Can you work these out from the model? Positions are in its coordinate system, mm. Face numbers are marked on the shaded views. Coordinates: 2 decimals unless noted, no trailing zeros. Loops run counter-clockwise (first coordinate to the right, second up) from the corner with the lowest first, then second, coordinate; pieces in that order, holes last. Notation, with made-up numbers: (37.5, 72) - (46.5, 72) arc R25 ccw to (46.5, 96) - close; hole circle Ø6 at (55, 32). An arc over 180 degrees is marked (long way). Put each result on its own line as item: value. Start each with the question number.
from build123d import *

# Parameters (mm, degrees)
SKETCH1_W           = 76.2
SKETCH1_H           = 31.75
BOSS_EXTRUDE1_DEPTH = 1.27
FILLET1_R           = 3.175
SKETCH2_W           = 68.58
SKETCH2_H           = 24.13
BOSS_EXTRUDE2_DEPTH = 1.27
SKETCH3_R           = 1.27
CUT_EXTRUDE1_DEPTH  = 42.353079994
CHAMFER1_SIZE       = 0.508


with BuildPart() as part:
    # Sketch1 → Boss-Extrude1 (new body)
    with BuildSketch(Plane(origin=(0, 0, 0), x_dir=(1, 0, 0), z_dir=(0, 1, 0))):
        Rectangle(SKETCH1_W, SKETCH1_H)
    extrude(amount=BOSS_EXTRUDE1_DEPTH)

    # Fillet1
    fillet1_edges = [part.edges().sort_by_distance(p)[0] for p in [
        (-38.1, 0.635, -15.875),
        (38.1, 0.635, -15.875),
        (38.1, 0.635, 15.875),
        (-38.1, 0.635, 15.875),
    ]]
    fillet(fillet1_edges, radius=FILLET1_R)

    # Sketch2 → Boss-Extrude2 (add)
    with BuildSketch(Plane(origin=(0, 1.27, 0), x_dir=(1, 0, 0), z_dir=(0, 1, 0))):
        with BuildLine():
            Line((34.925, 13.335), (-34.925, 13.335))
            ThreePointArc((-34.925, 13.335), (-35.374012806, 13.149012806), (-35.56, 12.7))
            Line((-35.56, 12.7), (-35.56, -12.7))
            ThreePointArc((-35.56, -12.7), (-35.374012806, -13.149012806), (-34.925, -13.335))
            Line((-34.925, -13.335), (34.925, -13.335))
            ThreePointArc((34.925, -13.335), (35.374012806, -13.149012806), (35.56, -12.7))
            Line((35.56, -12.7), (35.56, 12.7))
            ThreePointArc((35.56, 12.7), (35.374012806, 13.149012806), (34.925, 13.335))
        make_face()
        Rectangle(SKETCH2_W, SKETCH2_H, mode=Mode.SUBTRACT)
    extrude(amount=BOSS_EXTRUDE2_DEPTH)

    # Sketch3 → Cut-Extrude1 (cut, through all)
    with BuildSketch(Plane.XZ):
        with Locations(Location((34.925, -12.7, 0), (0, 0, 270))):
            Circle(SKETCH3_R)
        with Locations(Location((0, 12.7, 0), (0, 0, 270))):
            Circle(SKETCH3_R)
        with Locations(Location((-34.925, -12.7, 0), (0, 0, 270))):
            Circle(SKETCH3_R)
    extrude(amount=-CUT_EXTRUDE1_DEPTH, mode=Mode.SUBTRACT)

    # Chamfer1
    chamfer1_edges = [part.edges().sort_by_distance(p)[0] for p in [
        (-38.1, 0, 0),
        (0, 0, -15.875),
        (38.1, 0, 0),
        (0, 0, 15.875),
        (-37.17006403, 0, 14.94506403),
        (37.17006403, 0, 14.94506403),
        (37.17006403, 0, -14.94506403),
        (-37.17006403, 0, -14.94506403),
    ]]
    chamfer(chamfer1_edges, length=CHAMFER1_SIZE)


solid = part.part
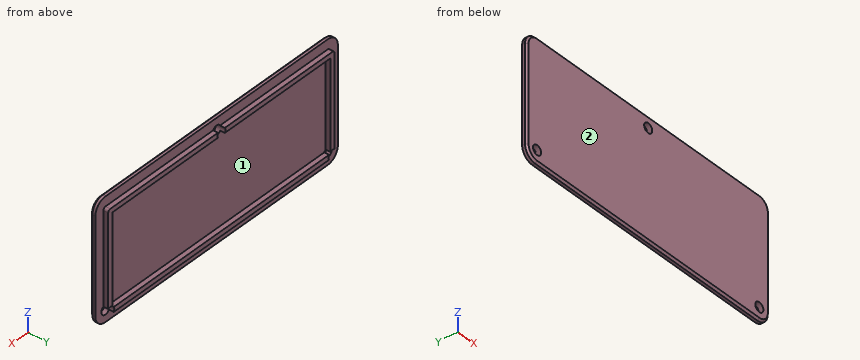
Q1. We'd pull the mould along X, two halves only. Please class the marked faces 1 and 2: released by +X, released by -X, zero draft, split by the parting line, or undercut.
Q2. I want a section at B-B on z = -1. List the corners of the cut face in (x, y) for me, and give its area (3 significant figures).
Q3. I want a section at A-A on x = 0. List the corners of the cut face in (y, z) for me (3 decimals), and give its area (3 significant figures).
Q4. Please list where these lines run through material, in increasing order: line 1 along Z through (x, y) = (3, 2.2) (3 decimals); line 2 along X through (y, z) = (1.45, -10.5); line 3 along X through (y, z) = (0.65, -12.7) (3 decimals). Write a range as [from, to].
Q5. Will these pins go through, and if not, where does the flat tip stop? pin 1 (1.4 mm diameter, centred on x = -15, y = 2, fed in from +Z) (3 decimals); pin 2 (1.4 mm diameter, centred on y = 2, z = 3.5, fed in from +X); pin 3 (0.6 mm diameter, centred on x = 12, y = 2, fed in from -Z) (3 decimals).
Calculated:
1. face 1: undercut
1. face 2: zero draft
2. outline: (-38.1, 0.51) - (-37.59, 0) - (37.59, 0) - (38.1, 0.51) - (38.1, 1.27) - (35.56, 1.27) - (35.56, 2.54) - (34.29, 2.54) - (34.29, 1.27) - (-34.29, 1.27) - (-34.29, 2.54) - (-35.56, 2.54) - (-35.56, 1.27) - (-38.1, 1.27) - close
2. area: 99.7 mm2
3. outline: (0, -15.367) - (0.508, -15.875) - (1.27, -15.875) - (1.27, -13.335) - (2.54, -13.335) - (2.54, -12.065) - (1.27, -12.065) - (1.27, 11.43) - (0, 11.43) - close; (0, 13.97) - (1.27, 13.97) - (1.27, 15.875) - (0.508, 15.875) - (0, 15.367) - close
3. area: 38.5 mm2
4. line 1: [-13.335, -12.065], [12.065, 13.335]
4. line 2: [-35.56, -34.29], [34.29, 35.56]
4. line 3: [-38.1, -36.195], [-33.655, 33.655], [36.195, 38.1]
5. pin 1: z = 13.335
5. pin 2: x = 35.56
5. pin 3: z = -13.335
